Autodesk Inventor part; units mm, degrees
ref_plane "YZ Plane" through (0, 0, 0) normal (1, 0, 0) x (0, 1, 0)
ref_plane "XZ Plane" through (0, 0, 0) normal (0, 1, 0) x (-1, 0, 0)
ref_plane "XY Plane" through (0, 0, 0) normal (0, 0, 1) x (1, 0, 0)
sketch "Sketch1" plane through (0, 0, 0) normal (0, 1, 0) x (-1, 0, 0)
  line L0 (0, 108) -> (0, 0)
  line L1 (0, 0) -> (10.412, 0)
  line L2 (10.412, 0) -> (80.1677, 18.691)
  line L3 (80.1677, 18.691) -> (80.1677, 89.309)
  line L4 (80.1677, 89.309) -> (10.412, 108)
  line L5 (10.412, 108) -> (0, 108)
  line L6 (2.5529, 107) -> (1, 101.2044) construction
  line L7 (1, 101.2044) -> (68.6148, 83.0871) construction
  line L8 (68.6148, 83.0871) -> (70.1677, 88.8827) construction
  line L9 (70.1677, 88.8827) -> (2.5529, 107) construction
  line L10 (1, 6.7956) -> (2.5529, 1) construction
  line L11 (2.5529, 1) -> (70.1677, 19.1173) construction
  line L12 (70.1677, 19.1173) -> (68.6148, 24.9129) construction
  line L13 (68.6148, 24.9129) -> (1, 6.7956) construction
  line L14 (71.1677, 88.309) -> (77.1677, 88.309) construction
  line L15 (77.1677, 88.309) -> (77.1677, 19.691) construction
  line L16 (77.1677, 19.691) -> (71.1677, 19.691) construction
  line L17 (71.1677, 19.691) -> (71.1677, 88.309) construction
  line L18 (17.0418, 103.1177) -> (15.4889, 97.3222)
  line L19 (15.4889, 97.3222) -> (23.2163, 95.2516)
  line L20 (23.2163, 95.2516) -> (24.7692, 101.0472)
  line L21 (24.7692, 101.0472) -> (17.0418, 103.1177)
  line L22 (47.9514, 94.8355) -> (46.3985, 89.0399)
  line L23 (46.3985, 89.0399) -> (54.1259, 86.9694)
  line L24 (54.1259, 86.9694) -> (55.6788, 92.765)
  line L25 (55.6788, 92.765) -> (47.9514, 94.8355)
  line L26 (15.4889, 10.6778) -> (17.0418, 4.8823)
  line L27 (17.0418, 4.8823) -> (24.7692, 6.9528)
  line L28 (24.7692, 6.9528) -> (23.2163, 12.7484)
  line L29 (23.2163, 12.7484) -> (15.4889, 10.6778)
  line L30 (46.3985, 18.9601) -> (47.9514, 13.1645)
  line L31 (47.9514, 13.1645) -> (55.6788, 15.235)
  line L32 (55.6788, 15.235) -> (54.1259, 21.0306)
  line L33 (54.1259, 21.0306) -> (46.3985, 18.9601)
  line L34 (54.9024, 89.8672) -> (69.3913, 85.9849) construction
  line L35 (16.2653, 7.7801) -> (1.7765, 3.8978) construction
  line L36 (54.9024, 18.1328) -> (69.3913, 22.0151) construction
  line L37 (16.2653, 100.2199) -> (1.7765, 104.1022) construction
  line L38 (71.1677, 80.309) -> (77.1677, 80.309)
  line L39 (77.1677, 80.309) -> (77.1677, 72.309)
  line L40 (77.1677, 72.309) -> (71.1677, 72.309)
  line L41 (71.1677, 72.309) -> (71.1677, 80.309)
  line L42 (71.1677, 35.691) -> (77.1677, 35.691)
  line L43 (77.1677, 35.691) -> (77.1677, 27.691)
  line L44 (77.1677, 27.691) -> (71.1677, 27.691)
  line L45 (71.1677, 27.691) -> (71.1677, 35.691)
  line L46 (74.1677, 80.309) -> (74.1677, 88.309) construction
  line L47 (74.1677, 27.691) -> (74.1677, 19.691) construction
  dimension "d0" = 70
  dimension "d1" = 6
  dimension "d3" = 70
  dimension "d4" = 6
  dimension "d7" = 3
  dimension "d8" = 3
  dimension "d9" = 6
  dimension "d10" = 3
  dimension "d11" = 1
  dimension "d12" = 1
  dimension "d13" = 1
  dimension "d14" = 1
  dimension "d15" = 15
  dimension "d16" = 1
  dimension "d17" = 1
  dimension "d18" = 1
  dimension "d19" = 108
  dimension "d20" = 8
  dimension "d21" = 15
  dimension "d22" = 8
extrude "Extrusion7" add sketch "Sketch1" along normal blind 6
sketch "Sketch7" plane through (0, 0, 0) normal (0, -1, 0) x (1, 0, 0)
  line L0 (0, 0) -> (0, 108)
  line L1 (0, 92) -> (-6, 92)
  line L2 (-6, 92) -> (-6, 76)
  line L3 (-6, 76) -> (0, 76)
  line L4 (0, 76) -> (0, 92)
  dimension "d74" = 16
  dimension "d75" = 16
  dimension "d76" = 6
extrude "Extrusion8" cut sketch "Sketch7" against normal blind 6
sketch "Sketch8" plane through (0, 0, 0) normal (0, -1, 0) x (1, 0, 0)
  line L0 (-77.1677, 72.309) -> (-71.1677, 35.691) construction
  line L1 (-77.1677, 35.691) -> (-71.1677, 72.309) construction
  circle A0 centre (-74.1677, 54) radius 2.25
  dimension "d80" = 4.5
extrude "Extrusion9" cut sketch "Sketch8" against normal blind 6
sketch "Sketch9" plane through (0, 0, 0) normal (0, -1, 0) x (1, 0, 0)
  line L0 (-46.3985, 18.9601) -> (-24.7692, 6.9528) construction
  line L1 (-23.2163, 12.7484) -> (-47.9514, 13.1645) construction
  circle A0 centre (-35.5839, 12.9564) radius 2.25
  dimension "d83" = 4.5
extrude "Extrusion10" cut sketch "Sketch9" against normal blind 6
sketch "Sketch10" plane through (0, 0, 0) normal (0, -1, 0) x (1, 0, 0)
  line L0 (0, 0) -> (0, 76)
  line L1 (0, 68.25) -> (0, 63.75)
  line L2 (-16.3, 63.75) -> (-16.3, 68.25)
  line L3 (-12.3, 70.75) -> (-5, 70.75)
  line L4 (-5, 61.25) -> (-12.3, 61.25)
  line L5 (-16.3, 68.25) -> (-12.3, 68.25)
  line L6 (-5, 68.25) -> (0, 68.25)
  line L7 (0, 63.75) -> (-5, 63.75)
  line L8 (-12.3, 63.75) -> (-16.3, 63.75)
  line L9 (-12.3, 61.25) -> (-12.3, 63.75)
  line L10 (-12.3, 68.25) -> (-12.3, 70.75)
  line L11 (-5, 70.75) -> (-5, 68.25)
  line L12 (-5, 63.75) -> (-5, 61.25)
  line L13 (0, 34.25) -> (0, 29.75)
  line L14 (-16.3, 29.75) -> (-16.3, 34.25)
  line L15 (-12.3, 36.75) -> (-5, 36.75)
  line L16 (-5, 27.25) -> (-12.3, 27.25)
  line L17 (-16.3, 34.25) -> (-12.3, 34.25)
  line L18 (-5, 34.25) -> (0, 34.25)
  line L19 (0, 29.75) -> (-5, 29.75)
  line L20 (-12.3, 29.75) -> (-16.3, 29.75)
  line L21 (-12.3, 27.25) -> (-12.3, 29.75)
  line L22 (-12.3, 34.25) -> (-12.3, 36.75)
  line L23 (-5, 36.75) -> (-5, 34.25)
  line L24 (-5, 29.75) -> (-5, 27.25)
  point P0 (0, 108)
  point P1 (-16.3, 66)
  point P2 (-16.3, 32)
  dimension "d86" = 4.5
  dimension "d87" = 2.5
  dimension "d88" = 2.5
  dimension "d89" = 5
  dimension "d90" = 7.3
  dimension "d91" = 4
  dimension "d92" = 4.5
  dimension "d93" = 2.5
  dimension "d94" = 2.5
  dimension "d95" = 5
  dimension "d96" = 7.3
  dimension "d97" = 4
  dimension "d98" = 42
  dimension "d99" = 34
extrude "Extrusion11" cut sketch "Sketch10" against normal blind 6
chamfer "Chamfer2" distance 2 angle 45 2 edges at (-80.1677, 3, 89.309) (-80.1677, 3, 18.691)
sketch "Sketch11" plane through (0, 0, 0) normal (0, -1, 0) x (1, 0, 0)
  line L0 (0, 0) -> (0, 29.75)
  line L1 (0, 34.25) -> (0, 63.75)
  line L2 (0, 92) -> (0, 108)
  line L3 (0, 108) -> (-10.412, 108)
  line L4 (0, 102) -> (4, 102)
  line L5 (6, 100) -> (6, 96)
  line L6 (4, 94) -> (0, 94)
  line L7 (0, 94) -> (0, 102)
  line L8 (0, 58) -> (4, 58)
  line L9 (6, 56) -> (6, 52)
  line L10 (4, 50) -> (0, 50)
  line L11 (0, 50) -> (0, 58)
  line L12 (0, 14) -> (4, 14)
  line L13 (6, 12) -> (6, 8)
  line L14 (4, 6) -> (0, 6)
  line L15 (0, 6) -> (0, 14)
  arc A0 (6, 100) -> (4, 102) centre (4, 100) ccw
  arc A1 (4, 94) -> (6, 96) centre (4, 96) ccw
  arc A2 (6, 56) -> (4, 58) centre (4, 56) ccw
  arc A3 (4, 50) -> (6, 52) centre (4, 52) ccw
  arc A4 (6, 12) -> (4, 14) centre (4, 12) ccw
  arc A5 (4, 6) -> (6, 8) centre (4, 8) ccw
  dimension "d105" = 2
  dimension "d106" = 8
  dimension "d107" = 8
  dimension "d108" = 8
  dimension "d109" = 6
  dimension "d110" = 6
  dimension "d111" = 36
  dimension "d112" = 36
extrude "Extrusion12" add sketch "Sketch11" against normal blind 6
equation "\"d3\" = d0"
equation "\"d4\" = d1"
equation "\"d8\" = d7"
equation "\"d9\" = d1"
equation "\"d10\" = d7"
equation "\"d12\" = d11"
equation "\"d88\" = d87"
equation "\"d94\" = d93"
properties part number "front_panel_2004_brace_right"
Could you check a few things on this model? Use its own coordinates, in mm. A direction names the side the tool comes from. Round coordinates to 2 decimals unless told otherwise and drop trailing zeros. Loops run counter-clockwise (first coordinate to the right, second up) from the corner with the lowest first, then second, coordinate; pieces in that order, holes last. Notation, with made-up numbers: (16.25, 83.25) - (42.25, 83.25) arc R12 ccw to (42.25, 99.25) - close; hole circle Ø7 at (25.5, 86.25). An arc over 180 degrees is marked (long way). Answer as CSV lines item,"result".
1. I want a section at B-B on x = -19.5. List the corners of the cut face in (y, z) for me, then the cut area to 3 significant figures.
Filled in:
outline,"(0, 2.44) - (6, 2.44) - (6, 5.54) - (0, 5.54) - close; (0, 11.75) - (6, 11.75) - (6, 96.25) - (0, 96.25) - close; (0, 102.46) - (6, 102.46) - (6, 105.56) - (0, 105.56) - close"
area,"544 mm^2"
2. We'd pull the mould along X, two halves only. Please class faces 1 (the face through (0, 3, 61)), 2 (the face through (-51.869, 2.958, 93.786)), 3 (the face through (-36, 0, 55)): +X half, -X half, draft (parallel to the pull), parting line (faces both ways), or undercut.
Filled in:
face 1,"+X half"
face 2,"undercut"
face 3,"draft"
3. For pin 1 Ø1.6 at (y, z) = (2.5, 92.5) entering from +X; pin 2 Ø2 at (x, y) = (-34.5, 1.5) entering from -Z; pin 3 Ø1.3 at (y, z) = (4, 32) entering from +X, each with a flat end and sliding along its axis, tell me the tip position at first contact or that it passes through.
Filled in:
pin 1,"stops at x = 0"
pin 2,"stops at z = 6.19"
pin 3,"stops at x = -16.3"
4. I want a section at D-D on z = 40. List the corners of the cut face in (x, y) for me, then the cut area to 3 significant figures.
Filled in:
outline,"(-80.17, 0) - (0, 0) - (0, 6) - (-80.17, 6) - close"
area,"481 mm^2"
5. Please list where these lines run through material, in increasing order: line 1 along Z through (x, y) = (-6.5, 5.4); line 2 along X through (y, z) = (1.85, 78.5); line 3 along Z through (x, y) = (-49, 1.15). Write a range as [from, to].
Filled in:
line 1,"z = [0, 27.25], [36.75, 61.25], [70.75, 108]"
line 2,"x = [-80.17, -77.17], [-71.17, -6]"
line 3,"z = [10.34, 13.45], [19.66, 88.34], [94.55, 97.66]"
6. On a 3-axis mill with a long thin cutter (end or side, diameter ignored), from which of +Z, -Z, +X, -X, +Y, -Y can I reach the whole of each face in a straight line? I mean faces 4 (the face through (-79.188, 2.958, 19.415)), 5 (the face through (-77.168, 3, 76)), 6 (the face through (-2, 3, 63.75)). Say none if no direction works.
Filled in:
face 4,"-Z, -X, +Y, -Y"
face 5,"+Y, -Y"
face 6,"+X, +Y, -Y"
7. I want a section at A-A on z = 54. List the corners of the cut face in (x, y) for me, then the cut area to 3 significant figures.
Filled in:
outline,"(-80.17, 0) - (-76.42, 0) - (-76.42, 6) - (-80.17, 6) - close; (-71.92, 0) - (6, 0) - (6, 6) - (-71.92, 6) - close"
area,"490 mm^2"
8. I want a section at C-C on y = 4.8. Count the separate pieces of the cut face and the enclosed holes in it, then the cut area to 3 significant figures.
Filled in:
separate pieces,"1"
enclosed holes,"8"
area,"6,850 mm^2"
